Read the model definition and answer for the solid it produces. Units are mm, in the model's axes. A direction names the side the tool comes from. Give positions to 0.01 mm unless a question says otherwise; leave off trailing zeros. Loops run counter-clockwise (first coordinate to the right, second up) from the corner with the lowest first, then second, coordinate; pieces in that order, holes last. Notation, with made-up numbers: (-6.5, -19) - (45.5, -19) arc R18 ccw to (45.5, -13) - close; hole circle Ø7 at (-28, 27). An arc over 180 degrees is marked (long way). Write each question's results on one line, items separated by ' | '. Start each with the question number.
Q1. The part is cut by section D-D, the plane y = 72. Write down the section's boundary in (x, z), plus the area to 3 significant figures.
Q2. Given pin 1 (1 mm diameter, centred on x = -981, z = -197, fed in from -Y); pin 2 (1 mm diameter, centred on x = -972, y = 74.5, fed in from +Z); pin 3 (21 mm diameter, centred on x = -978.11, z = -277.95, fed in from -Y), each flat-ended and moving along its own axis, determine where each tip first touches the part or whether it passes through.
Q3. Determine the mould class of faces 1 (the flat face through (-978, 105, -195.872)), 2 (the flat face through (-978, 115.108, -268)), 3 (the flat face through (-978, 113.108, -267)), 4 (the flat face through (-982, 107, -337.707)) for opening direction Z: +Z half, -Z half, draft (parallel to the pull), parting line (faces both ways), or undercut.
Q4. Find the intervals of material crossed by line 1 (Z direction, x = -966.5, y = 109); line 2 (Z direction, x = -991, y = 67); line 3 (Y direction, x = -992, z = -292), in increasing order. Write a range as from..to.
Q5. The part is cut by section C-C, the plane z = -226. Write down the section's boundary in (x, y).
Q6. The part is cut by section A-A, the plane x = -980. State how many separate pieces and enclosed holes the cut face has, plus the area to 3 significant figures.
Q7. For faces 5 (the cylindrical face through (-984.45, 114.09, -225.04)), 6 (the flat face through (-978, 104, -197.878)), determine the directions among +Z, -Z, +X, -X, +Y, -Y from which every point of the face is accessible in a straight line to the end or side of a thin tool.
Autodesk Inventor part; units mm, degrees
ref_plane "YZ Plane" through (0, 0, 0) normal (1, 0, 0) x (0, 1, 0)
ref_plane "XZ Plane" through (0, 0, 0) normal (0, 1, 0) x (-1, 0, 0)
ref_plane "XY Plane" through (0, 0, 0) normal (0, 0, 1) x (1, 0, 0)
ref_plane "Plano de trabalho5" through (-1094.0332, 113.1084, -225.312) normal (0, 1, 0) x (1, 0, 0)
sketch "Esboço10" plane through (-1094.0332, 113.1084, -225.312) normal (0, 1, 0) x (1, 0, 0)
  line L0 (115.9279, 81.534) -> (115.9279, 81.534)
  circle A0 centre (115.9279, -5.1435) radius 8.001
  circle A1 centre (115.9279, 52.6415) radius 8.001
  line L1 (98.0571, -16.7405) -> (133.6171, -16.7405)
  line L2 (133.6171, 68.072) -> (133.6171, 42.672)
  line L3 (133.6171, -16.7405) -> (98.0571, -16.7405)
  line L4 (98.0571, -16.7405) -> (98.0571, 99.695)
  line L5 (133.6171, 99.695) -> (133.6171, -16.7405)
  line L6 (98.0571, 99.695) -> (98.0571, 110.395)
  line L7 (98.0571, 110.395) -> (133.6171, 110.395)
  line L8 (133.6171, 110.395) -> (133.6171, 99.695)
  line L9 (133.6171, 110.395) -> (98.0571, 110.395)
  line L10 (98.0571, 110.395) -> (98.0571, -16.7405)
  line L11 (98.0571, -16.7405) -> (133.6171, -16.7405)
  line L12 (133.6171, -16.7405) -> (133.6171, 110.395)
  point P0 (1094.0332, -225.312)
  dimension "d30" = 0
  dimension "d35" = 16.002
  dimension "d37" = 16.002
  dimension "d65" = 10.7
extrude "Extrusão9" add sketch "Esboço10" along normal blind 2
sketch "Esboço14" plane through (-960.416, 113.1084, -335.707) normal (0, 0, -1) x (-1, 0, 0)
  line L0 (0, 2) -> (35.56, 2)
  line L1 (35.56, 2) -> (35.56, -18.1014)
  line L2 (0, -5.2428) -> (35.56, -18.1014)
  line L3 (0, -5.2428) -> (0, 2)
  point P0 (-960.416, -113.1084)
extrude "Extrusão12" add sketch "Esboço14" along normal blind 2
sketch "Esboço15" plane through (-960.416, 113.1084, -335.707) normal (0, 0, 1) x (1, 0, 0)
  line L0 (-35.56, -18.1014) -> (-35.56, 2)
  line L1 (0, 2) -> (0, -5.2428)
  line L2 (-35.56, -18.1014) -> (0, -5.2428)
  line L3 (0, -5.2428) -> (0, -18.1014)
  line L4 (0, -18.1014) -> (-35.56, -18.1014)
  point P0 (960.416, -113.1084)
extrude "Extrusão13" add sketch "Esboço15" against normal blind 2.0066
sketch "Esboço16" plane through (-960.416, 113.1084, -335.707) normal (0, 0, 1) x (1, 0, 0)
  line L0 (-35.56, -18.1014) -> (-35.56, 2)
  line L1 (-35.56, -18.1014) -> (0, -18.1014)
  line L2 (0, -18.1014) -> (0, -56.2014)
  line L3 (0, -56.2014) -> (-35.56, -56.2014)
  line L4 (-35.56, -56.2014) -> (-35.56, -18.1014)
  point P0 (960.416, -113.1084)
  dimension "d70" = 38.1
extrude "Extrusão14" add sketch "Esboço16" against normal blind 2.0066
sketch "Esboço17" plane through (-995.976, 113.1084, -208.5715) normal (0, 0, 1) x (1, 0, 0)
  line L0 (35.56, 0) -> (35.56, 2)
  line L1 (0, 0) -> (0, 2)
  line L2 (35.56, 0) -> (0, 0)
  line L3 (0, 0) -> (0, 2)
  line L4 (0, 2) -> (35.56, 2)
  line L5 (35.56, 2) -> (35.56, 0)
  point P0 (995.976, -113.1084)
extrude "Extrusão15" add sketch "Esboço17" along normal blind 12.7
sketch "Esboço18" plane through (-1094.0332, 113.1084, -225.312) normal (0, -1, 0) x (1, 0, 0)
  line L0 (98.0571, 29.4405) -> (133.6171, 29.4405)
  line L1 (133.6171, 29.4405) -> (133.6171, -110.395)
  line L2 (98.0571, 29.4405) -> (133.6171, 29.4405)
  line L3 (133.6171, 29.4405) -> (133.6171, 27.4339)
  line L4 (133.6171, 27.4339) -> (98.0571, 27.4339)
  line L5 (98.0571, 27.4339) -> (98.0571, 29.4405)
  point P0 (1094.0332, 225.312)
  dimension "d75" = 2.0066
extrude "Extrusão16" add sketch "Esboço18" along normal blind 17.9832
properties part number "Fixação sem Tanque_2 - DIN"
Check sheet entries:
1) outline: (-995.98, -337.71) - (-960.42, -337.71) - (-960.42, -335.71) - (-995.98, -335.71) - close | area: 71.4 mm^2
2) pin 1: stops at y = 95.13 | pin 2: stops at z = -335.71 | pin 3: stops at y = 113.11
3) face 1: +Z half | face 2: draft | face 3: undercut | face 4: -Z half
4) line 1: z = -337.71..-335.71, -197.88..-195.87 | line 2: z = -337.71..-335.71 | line 3: y = 113.11..115.11
5) outline: (-995.98, 113.11) - (-983.58, 113.11) - (-983.58, 115.11) - (-995.98, 115.11) - close; (-972.63, 113.11) - (-960.42, 113.11) - (-960.42, 115.11) - (-972.63, 115.11) - close
6) separate pieces: 3 | enclosed holes: 0 | area: 370 mm^2
7) face 5: +Y, -Y | face 6: +X, -X, -Y
